For this review, take the finished solid that the model builds, in its own axes (mm). A direction names the side the tool comes from. Round coordinates to 2 decimals unless told otherwise and drop trailing zeros. Write each loop counter-clockwise with the first axis right and the second up, starting at its lowest first coordinate (ties: lowest second). Pieces come first, ordered by that corner, then holes. Notation, with made-up numbers: (57.25, 19) -> (112.25, 19) arc R34 ccw to (112.25, 54) -> close; hole circle Ø7 at (-2, 34.25). An arc over 180 degrees is marked (long way). Write each question's results on one line, items separated by ' | '. Start each with the question number.
Item 1: Add section B-B (z = 38). State the section outline as (x, y) points, plus the area to 3 significant figures.
Item 2: Add section A-A (x = 12.7). State the section outline as (y, z) points.
Item 3: Clearance check with flat-ended pins moving along their axes: pin 1 (10 mm diameter, centred on x = 79, y = -7.5, fed in from +Z); pin 2 (7 mm diameter, centred on x = 10.5, y = -1, fed in from +Z); pin 3 (1.5 mm diameter, centred on y = -12, z = 30.5, fed in from +X). State where each tip first meets the part, or that it passes through.
Item 4: Add section C-C (y = -21.5). State the section outline as (x, z) points (1 decimal).
Item 5: Tool access review of faces 1 (the flat face through (13, 0, 27.94)), 2 (the flat face through (0, 0, 33)), 3 (the flat face through (25.4, 0, 63)): name each direction out of +Z, -Z, +X, -X, +Y, -Y from which nothing blocks a thin tool from reaching the whole face with its end or side.
Item 6: To check wall thickness, follow line 1 along Y through (x, z) = (12.7, 43); line 2 along X through (y, z) = (18.5, 62.5); line 3 along Z through (x, y) = (83.5, 14) (3 decimals). State the ranges of each line that lie inside material, in increasing order.
Item 7: Add section D-D (z = 13). State the section outline as (x, y) points, plus the area to 3 significant figures.
Item 8: The part is to be moulded in two halves that separate along Y. For faces 4 (the flat face through (55.6, 6.6, 46.1)), 5 (the cylindrical face through (7.439, 4.824, 47.257)), 6 (the flat face through (83.517, -12.143, 25.175)), say which applies: +Y half, -Y half, draft (parallel to the pull), parting line (faces both ways), or undercut.
from build123d import *

# Parameters (mm, degrees)
F1_DEPTH = 31.75
F2_R     = 7.1374
F3_DEPTH = 38.1
F8_DEPTH = 47.0227251518


with BuildPart() as f1:
    # F0 (on Front) → F1 (new body, symmetric)
    with BuildSketch(Plane.XZ):
        Polygon((0, 66.04), (0, 0), (101.6, 0), (101.6, 25.4), (25.4, 59.69), (25.4, 66.04), align=None)
    extrude(amount=F1_DEPTH, both=True)

    # F2 (on face) → F3 (cut)
    with BuildSketch(Plane.XY.offset(66.04)):
        with Locations((12.7, 0)):
            Circle(F2_R)
    extrude(amount=-F3_DEPTH, mode=Mode.SUBTRACT)

    # F7 (on 3pt) → F8 (cut, through all)
    with BuildSketch(Plane(origin=(44.0556400507, -25.9150823828, 51.8301647655), x_dir=(0.79606128, 0.2706608352, -0.5413216704), z_dir=(0.6052160263, -0.3560094273, 0.7120188545))):
        Polygon((72.2863445278, -28.3980633142), (72.2863445278, 28.3980633142), (-7.4813839092, -4.2597094971), align=None)
    extrude(amount=F8_DEPTH, mode=Mode.SUBTRACT)


solid = f1.part
Responses:
1) outline: (0, -31.75) -> (56.89, -31.75) -> (73.6, -3.35) -> (73.6, 31.75) -> (0, 31.75) -> close; hole circle Ø14.27 at (12.7, 0) | area: 4,280 mm^2
2) outline: (-31.75, 0) -> (31.75, 0) -> (31.75, 66.04) -> (7.14, 66.04) -> (7.14, 27.94) -> (-7.14, 27.94) -> (-7.14, 66.04) -> (-31.75, 66.04) -> close
3) pin 1: stops at z = 36.27 | pin 2: stops at z = 27.94 | pin 3: stops at x = 78.32
4) outline: (0, 0) -> (101.6, 0) -> (101.6, 5.1) -> (50.9, 48.2) -> (25.4, 59.7) -> (25.4, 66) -> (0, 66) -> close
5) face 1: +Z | face 2: +Z, -Z, -X, +Y, -Y | face 3: +Z, +X, +Y, -Y
6) line 1: y = -31.75 to -7.14, 7.14 to 31.75 | line 2: x = 0 to 25.4 | line 3: z = 0 to 33.545
7) outline: (0, -31.75) -> (86.31, -31.75) -> (101.6, -5.75) -> (101.6, 31.75) -> (0, 31.75) -> close | area: 6,250 mm^2
8) face 4: draft | face 5: undercut | face 6: -Y half
